```python
from build123d import *

# Parameters (mm, degrees)
F0_R     = 10
F1_DEPTH = 1000
F2_R     = 10
F2_R_2   = 6
F3_DEPTH = 20
F4_R     = 10
F4_R_2   = 7.5
F5_DEPTH = 40
F6_R     = 10
F6_R_2   = 7.5
F7_DEPTH = 12
F8_W     = 1.15
F8_H     = 0.35


with BuildPart() as f1:
    # F0 (on Right) → F1 (new body)
    with BuildSketch(Plane.YZ):
        Circle(F0_R)
    extrude(amount=-F1_DEPTH)

    # F2 (on face) → F3 (cut)
    with BuildSketch(Plane.YZ):
        Circle(F2_R)
        Circle(F2_R_2, mode=Mode.SUBTRACT)
    extrude(amount=-F3_DEPTH, mode=Mode.SUBTRACT)

    # F4 (on face) → F5 (cut)
    with BuildSketch(Plane.YZ.offset(-20)):
        Circle(F4_R)
        Circle(F4_R_2, mode=Mode.SUBTRACT)
    extrude(amount=-F5_DEPTH, mode=Mode.SUBTRACT)

    # F6 (on face) → F7 (cut)
    with BuildSketch(Plane(origin=(-1000, 0, 0), x_dir=(0, -1, 0), z_dir=(-1, 0, 0))):
        Circle(F6_R)
        Circle(F6_R_2, mode=Mode.SUBTRACT)
    extrude(amount=-F7_DEPTH, mode=Mode.SUBTRACT)

    # F8 (on Front) → F9 (revolve, cut)
    with BuildSketch(Plane.XZ):
        with Locations((-997.575, 7.325)):
            Rectangle(F8_W, F8_H)
    revolve(axis=Axis((-986.6362512112, 0, 0), (1, 0, 0)), mode=Mode.SUBTRACT)


solid = f1.part
```
Geometry: final body of the model. Coordinates: model frame, mm. A direction names the side the tool comes from. Round coordinates to 2 decimals unless told otherwise and drop trailing zeros. Write each loop counter-clockwise with the first axis right and the second up, starting at its lowest first coordinate (ties: lowest second). Pieces come first, ordered by that corner, then holes. Notation, with made-up numbers: (-23, 49) -> (36, 49) arc R5 cw to (36, 58) -> close; hole circle Ø9 at (31, -10). An arc over 180 degrees is marked (long way). Return JSON: item names as keys, results as strings.
Q1. Set-up query: faces 1 (the flat face through (-60, 4, 7)), 2 (the cylindrical face through (-517.5, -2.17, -9.76)), 3 (the flat face through (-988, -4, 7)). Return all of +Z, -Z, +X, -X, +Y, -Y with unobstructed straight access to the full face (end or side cutting, diameter ignored); none if empty.
From the geometry:
{"face 1": "+X", "face 2": "+X, -X", "face 3": "-X"}
Q2. Ray query, line 1 (X direction, y = 6.75, z = 4); line 2 (Y direction, x = -549.5, z = 6.5); line 3 (Y direction, x = -158, z = 1.75). Return the intervals inside material, ascending.
From the geometry:
{"line 1": "-988 to -60", "line 2": "-7.6 to 7.6", "line 3": "-9.85 to 9.85"}
Q3. Section A-A on z = 0. Return the cut outline in (x, y), and give its area (3 significant figures).
From the geometry:
{"outline": "(-1000, -7.5) -> (-998.15, -7.5) -> (-998.15, -7.15) -> (-997, -7.15) -> (-997, -7.5) -> (-988, -7.5) -> (-988, -10) -> (-60, -10) -> (-60, -7.5) -> (-20, -7.5) -> (-20, -6) -> (0, -6) -> (0, 6) -> (-20, 6) -> (-20, 7.5) -> (-60, 7.5) -> (-60, 10) -> (-988, 10) -> (-988, 7.5) -> (-997, 7.5) -> (-997, 7.15) -> (-998.15, 7.15) -> (-998.15, 7.5) -> (-1000, 7.5) -> close", "area": "19,600 mm2"}
Q4. First-contact query: pin 1 Ø3 at (x, z) = (-324.5, 6) entering from +Y; pin 2 Ø5 at (x, z) = (-354, 3) entering from -Y; pin 3 Ø1 at (y, z) = (6.5, -6) entering from -X. Flat tips, straight axial feed; report the tip coordinate or a pass-through.
From the geometry:
{"pin 1": "y = 8.93", "pin 2": "y = -9.99", "pin 3": "x = -988"}
Q5. Section C-C on x = -236.5. Return the cut outline in (y, z).
From the geometry:
{"outline": "circle Ø20 at (0, 0)"}
